from build123d import *

# Parameters (mm, degrees)
IZIM1_W                     = 100
IZIM1_H                     = 56
IZIM1_R                     = 9.5
Y_KSEKLIK_EKSTR_ZYON1_DEPTH = 8
IZIM2_R                     = 2.6
KES_EKSTR_ZYON1_DEPTH       = 10


with BuildPart() as part:
    # Çizim1 → Yükseklik-Ekstrüzyon1 (new body)
    with BuildSketch(Plane.XY):
        with Locations((-2.031053151, 0.257686676)):
            Rectangle(IZIM1_W, IZIM1_H)
        with Locations((-32.031053151, 3.257686676)):
            Circle(IZIM1_R, mode=Mode.SUBTRACT)
        with Locations((27.968946849, 3.257686676)):
            Circle(IZIM1_R, mode=Mode.SUBTRACT)
        with Locations((-2.031053151, 3.257686676)):
            Circle(IZIM1_R, mode=Mode.SUBTRACT)
    extrude(amount=Y_KSEKLIK_EKSTR_ZYON1_DEPTH)

    # Çizim2 → Kes-Ekstrüzyon1 (cut)
    with BuildSketch(Plane(origin=(0, 0, 0), x_dir=(-1, 0, 0), z_dir=(0, 0, -1))):
        with Locations((-37.968946849, 20.757686676)):
            Circle(IZIM2_R)
        with Locations((-37.968946849, -12.242313324)):
            Circle(IZIM2_R)
        with Locations((42.031053151, -12.242313324)):
            Circle(IZIM2_R)
        with Locations((42.031053151, 20.757686676)):
            Circle(IZIM2_R)
    extrude(amount=-KES_EKSTR_ZYON1_DEPTH, mode=Mode.SUBTRACT)


solid = part.part
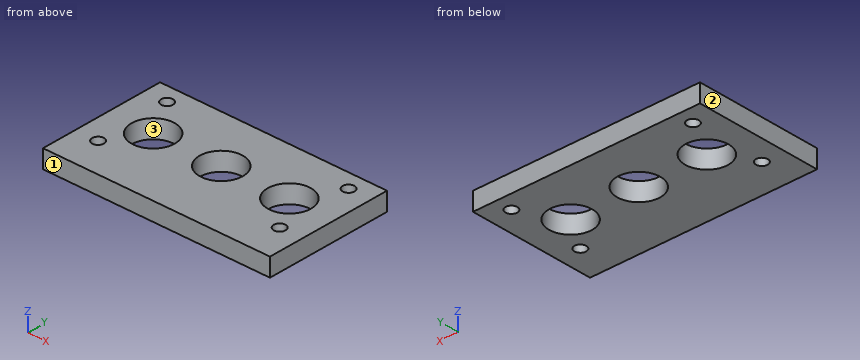
The model under review builds one solid part; all positions refer to its coordinate system, in mm. Face numbers are marked on the shaded views. Round coordinates to 2 decimals unless told otherwise and drop trailing zeros. Write each loop counter-clockwise with the first axis right and the second up, starting at its lowest first coordinate (ties: lowest second). Pieces come first, ordered by that corner, then holes. Notation, with made-up numbers: M 10,-25 L 23,-25 A18 ccw 23,-17 Z; hole C -3.5,40.25 d3. An arc over 180 degrees is marked long. Use a Markdown table: item, result. Add a question column.
Q1. The part is to be moulded in two halves that separate along Y. For the marked faces 1, 2 and 3, say which applies: pulls with the +Y half, pulls with the -Y half, needs draft (parallel to the pull), parting line crosses it, or undercut.
Q2. We need section B-B, the plane y = 19.5. State the section outline as (x, z) points, plus the area to 3 significant figures.
Q3. We need section C-C, the plane z = 2.5. State the section outline as (x, y) points.
Q4. We need section D-D, the plane x = 24.5. State the section outline as (y, z) points.
Q5. To check wall thickness, follow line 1 (X direction, y = 21, z = 3.75); line 2 (X direction, y = -10, z = 4); line 3 (Y direction, x = -32, z = 1.5). State the ranges of each line that lie inside material, in increasing order.
Q6. We need section A-A, the plane x = -23.5. State the section outline as (y, z) points, plus the area to 3 significant figures.
Q7. Insertion check: pin 1 (11.5 mm diameter, centred on x = -32.03, y = 3.26, fed in from -Z). The pin has a flat end and moves straight along its axis. Give the tip position at first contact, or say it passes through.
Findings below:
| question | item | result |
|---|---|---|
| 1 | face 1 | pulls with the -Y half |
| 1 | face 2 | needs draft |
| 1 | face 3 | undercut |
| 2 | outline | M -52.03,0 L -44.31,0 L -44.31,8 L -52.03,8 Z; M -39.76,0 L 35.69,0 L 35.69,8 L -39.76,8 Z; M 40.24,0 L 47.97,0 L 47.97,8 L 40.24,8 Z |
| 2 | area | 727 mm² |
| 3 | outline | M -52.03,-27.74 L 47.97,-27.74 L 47.97,28.26 L -52.03,28.26 Z; hole C -42.03,-12.24 d5.2; hole C -42.03,20.76 d5.2; hole C -32.03,3.26 d19; hole C -2.03,3.26 d19; hole C 27.97,3.26 d19; hole C 37.97,-12.24 d5.2; hole C 37.97,20.76 d5.2 |
| 4 | outline | M -27.74,0 L -5.59,0 L -5.59,8 L -27.74,8 Z; M 12.1,0 L 28.26,0 L 28.26,8 L 12.1,8 Z |
| 5 | line 1 | x = -52.03 to -44.62, -39.44 to 35.38, 40.56 to 47.97 |
| 5 | line 2 | x = -52.03 to -43.35, -40.71 to 36.65, 39.29 to 47.97 |
| 5 | line 3 | y = -27.74 to -6.24, 12.76 to 28.26 |
| 6 | outline | M -27.74,0 L -0.92,0 L -0.92,8 L -27.74,8 Z; M 7.44,0 L 28.26,0 L 28.26,8 L 7.44,8 Z |
| 6 | area | 381 mm² |
| 7 | pin 1 | passes through |
